from build123d import *

# Parameters (mm, degrees)
SKETCH_1_R                 = 4.1
SKETCH_1_R_2               = 1.6
SKETCH_1_R_3               = 1.7
F_10_CAMERA_SIDE_EAR_DEPTH = 5


with BuildPart() as part:
    # Эскиз1 → 10_Camera_side_ear (new body)
    with BuildSketch(Plane.XY):
        Polygon((-33, 0), (33, 0), (33, 24), (20, 45), (-20, 45), (-33, 24), align=None)
        with Locations((0, 24)):
            Circle(SKETCH_1_R, mode=Mode.SUBTRACT)
        with Locations((-9, 24)):
            Circle(SKETCH_1_R_2, mode=Mode.SUBTRACT)
        with Locations((9, 24)):
            Circle(SKETCH_1_R_2, mode=Mode.SUBTRACT)
        with Locations((0, 16)):
            Circle(SKETCH_1_R_2, mode=Mode.SUBTRACT)
        with Locations((0, 34)):
            Circle(SKETCH_1_R_2, mode=Mode.SUBTRACT)
        with Locations((-24, 8)):
            Circle(SKETCH_1_R_3, mode=Mode.SUBTRACT)
        with Locations((24, 8)):
            Circle(SKETCH_1_R_3, mode=Mode.SUBTRACT)
    extrude(amount=F_10_CAMERA_SIDE_EAR_DEPTH)


solid = part.part
CAD build for the part. Positions are in the model's coordinates, mm. Round coordinates to 2 decimals unless told otherwise and drop trailing zeros. Write each loop counter-clockwise with the first axis right and the second up, starting at its lowest first coordinate (ties: lowest second). Pieces come first, ordered by that corner, then holes. Notation, with made-up numbers: (-33, -20) -> (-7, -20) arc R20 cw to (-7, -8) -> close; hole circle Ø4 at (-34.75, 78). An arc over 180 degrees is marked (long way). Answer as a JSON object with one key per item and string values.
(1) Probe probe 1 along Y at (x, z) = (0, 1.6); probe 2 along X at (y, z) = (7, 1.5); probe 3 along Y at (x, z) = (-9, 3.9). List the from-to ranges inside material, lowest first. Write a range as [from, to].
Reported:
{"probe 1": "y = [0, 14.4], [17.6, 19.9], [28.1, 32.4], [35.6, 45]", "probe 2": "x = [-33, -25.37], [-22.63, 22.63], [25.37, 33]", "probe 3": "y = [0, 22.4], [25.6, 45]"}
(2) Pin check, flat tip, straight feed: P1, Ø3, axis at x = 0, y = 34, coming from the -Z side. Stop position of the tip, or through.
Reported:
{"P1": "passes through"}
(3) Two-plate mould, pull along X, no slides. Class faces 1 (the face through (-0.208, 17.586, 2.465)), 2 (the face through (0, 18, 0)), 3 (the face through (33, 12, 2)), 4 (the face through (-26.409, 34.647, 2.465)): +X half, -X half, draft (parallel to the pull), parting line (faces both ways), or undercut.
Reported:
{"face 1": "undercut", "face 2": "draft", "face 3": "+X half", "face 4": "-X half"}
(4) Band-saw the part on D-D, the plane z = 1.6. List the corners of the cut face in (x, y), then the cut area to 3 significant figures.
Reported:
{"outline": "(-33, 0) -> (33, 0) -> (33, 24) -> (20, 45) -> (-20, 45) -> (-33, 24) -> close; hole circle Ø3.4 at (-24, 8); hole circle Ø3.2 at (-9, 24); hole circle Ø8.2 at (0, 24); hole circle Ø3.2 at (0, 16); hole circle Ø3.2 at (0, 34); hole circle Ø3.2 at (9, 24); hole circle Ø3.4 at (24, 8)", "area": "2,590 mm^2"}
(5) Band-saw the part on B-B, the plane x = -9. List the corners of the cut face in (y, z).
Reported:
{"outline": "(0, 0) -> (22.4, 0) -> (22.4, 5) -> (0, 5) -> close; (25.6, 0) -> (45, 0) -> (45, 5) -> (25.6, 5) -> close"}
(6) Band-saw the part on A-A, the plane y = 16. List the corners of the cut face in (x, z), then the cut area to 3 significant figures.
Reported:
{"outline": "(-33, 0) -> (-1.6, 0) -> (-1.6, 5) -> (-33, 5) -> close; (1.6, 0) -> (33, 0) -> (33, 5) -> (1.6, 5) -> close", "area": "314 mm^2"}
(7) Band-saw the part on C-C, the plane y = 8. List the corners of the cut face in (x, z), then the cut area to 3 significant figures.
Reported:
{"outline": "(-33, 0) -> (-25.7, 0) -> (-25.7, 5) -> (-33, 5) -> close; (-22.3, 0) -> (22.3, 0) -> (22.3, 5) -> (-22.3, 5) -> close; (25.7, 0) -> (33, 0) -> (33, 5) -> (25.7, 5) -> close", "area": "296 mm^2"}
